Check sheet for the drawn part. Datum: minimum x, y, z corner. Units: mm. A direction names the side the tool comes from. Give positions to 0.01 mm unless a question says otherwise; leave off trailing zeros. Write each loop counter-clockwise with the first axis right and the second up, starting at its lowest first coordinate (ties: lowest second). Pieces come first, ordered by that corner, then holes. Notation, with made-up numbers: (59.5, 76) -> (109.5, 76) arc R13 cw to (109.5, 86) -> close; hole circle Ø4 at (45.25, 16.25). An arc over 180 degrees is marked (long way). Answer as CSV lines item,"result". Start each with the question number.
1) Tool access check on the marked faces 1 and 2. Record the directions out of +Z, -Z, +X, -X, +Y, -Y that give a thin tool (end or side, any length) a straight path to the whole face; none if there is none.
2) Gauge pin test, flat ends, axial feed: pin 1 Ø7.5 at (x, y) = (24, 43) entering from +Z; pin 2 Ø12 at (x, y) = (19.5, 30) entering from +Z; pin 3 Ø24 at (x, z) = (19, 51.5) entering from +Y. Record the tip position at first contact, or that the pin passes through.
3) Sectioned sample at C-C on y = 58. Record the cut outline in (x, z).
4) Sectioned sample at A-A on x = 3.5. Record the cut outline in (y, z), and give its area (3 significant figures).
5) Sectioned sample at B-B on z = 32.5. Record the cut outline in (x, y), and give its area (4 significant figures).
6) Material ranges on L1, parallel to Y at x = 9.5, z = 35; L2, parallel to Y at x = 33, z = 64.5; L3, parallel to Z at x = 21.5, y = 52.5, recorded low to high.
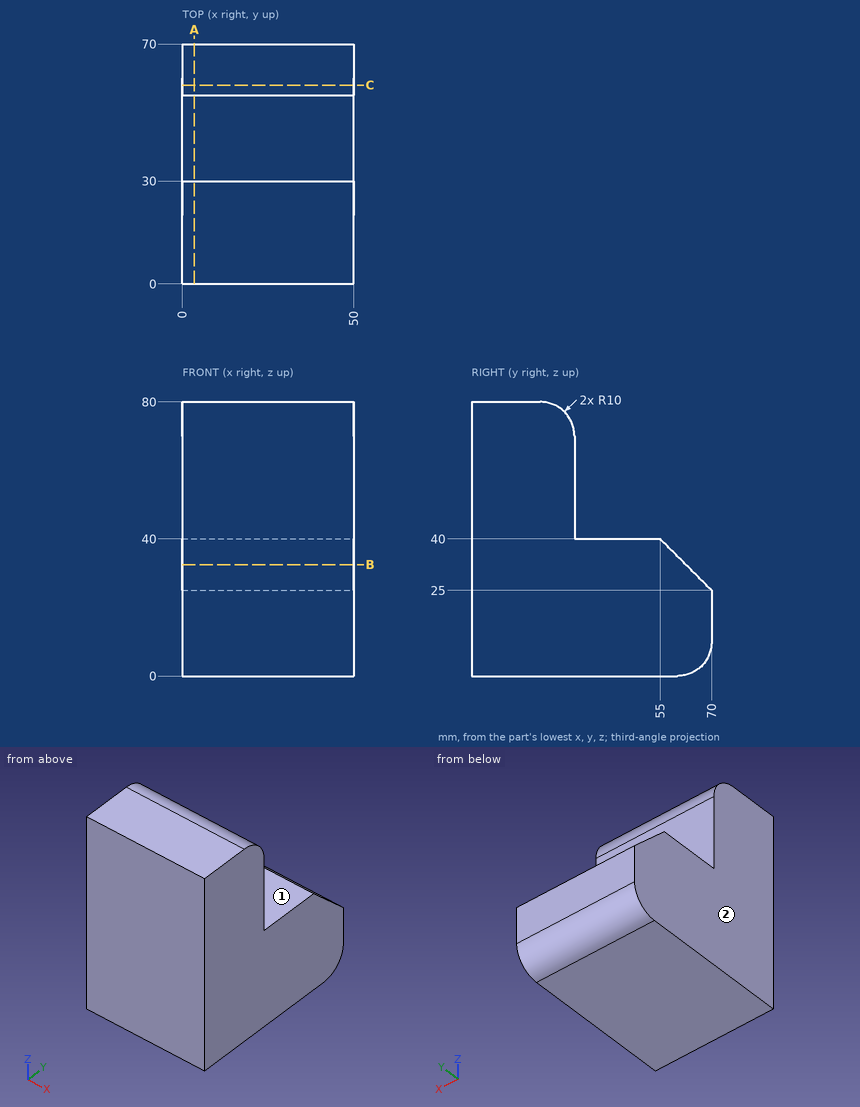
Ans:
1,face 1,"+Z, +X, -X, +Y"
1,face 2,"+Z, -Z, -X, +Y, -Y"
2,pin 1,"stops at z = 40"
2,pin 2,"stops at z = 79.17"
2,pin 3,"stops at y = 55.5"
3,outline,"(0, 0) -> (50, 0) -> (50, 37) -> (0, 37) -> close"
4,outline,"(0, 0) -> (60, 0) arc R10 ccw to (70, 10) -> (70, 25) -> (55, 40) -> (30, 40) -> (30, 70) arc R10 ccw to (20, 80) -> (0, 80) -> close"
4,area,"3,840 mm²"
5,outline,"(0, 0) -> (50, 0) -> (50, 62.5) -> (0, 62.5) -> close"
5,area,"3,125 mm²"
6,L1,"y = 0 to 60"
6,L2,"y = 0 to 30"
6,L3,"z = 0 to 40"
